Job drawing, mm, ordinate dimensions from the low corner. One solid piece. A direction names the side the tool comes from. Round coordinates to 2 decimals unless told otherwise and drop trailing zeros. Loops run counter-clockwise (first coordinate to the right, second up) from the corner with the lowest first, then second, coordinate; pieces in that order, holes last. Notation, with made-up numbers: M 10,32 L 50,32 A27 cw 50,59 Z; hole C -7.5,-4.5 d2. An arc over 180 degrees is marked long. Use a Markdown table: item, result. Add a question column.
(1) Band-saw the part on A-A, the plane y = 12.25. Write the cut outline in (x, z).
(2) Band-saw the part on B-B, the plane x = 7. Write the cut outline in (y, z) (1 decimal).
(3) Which spindle directions (+Z, -Z, +X, -X, +Y, -Y) get a long thin tool onto all of the face, cutting with end or side? Do the marked faces 1, 2 and 3. Say none if no direction does.
(4) Flat gauge pins, fed straight in: P1, Ø2, axis at y = 2.5, z = 7, coming from the -X side; P2, Ø8, axis at x = 5, y = 6, coming from the -Z side; P3, Ø5, axis at y = 8, z = 11.5, coming from the -X side. Where does each tip first touch, or does it go through?
(5) Band-saw the part on C-C, the plane z = 7. Write the cut outline in (x, y) (1 decimal), and give its area (3 significant figures).
(6) Band-saw the part on D-D, the plane y = 1.5. Write the cut outline in (x, z) (1 decimal), and give its area (3 significant figures).
(7) Wall check: L1, parallel to X at y = 2, z = 7; L2, parallel to Y at x = 9, z = 8.75; L3, parallel to Z at x = 2, y = 2.75 (1 decimal). Give the ranges that are in metal, low to high.
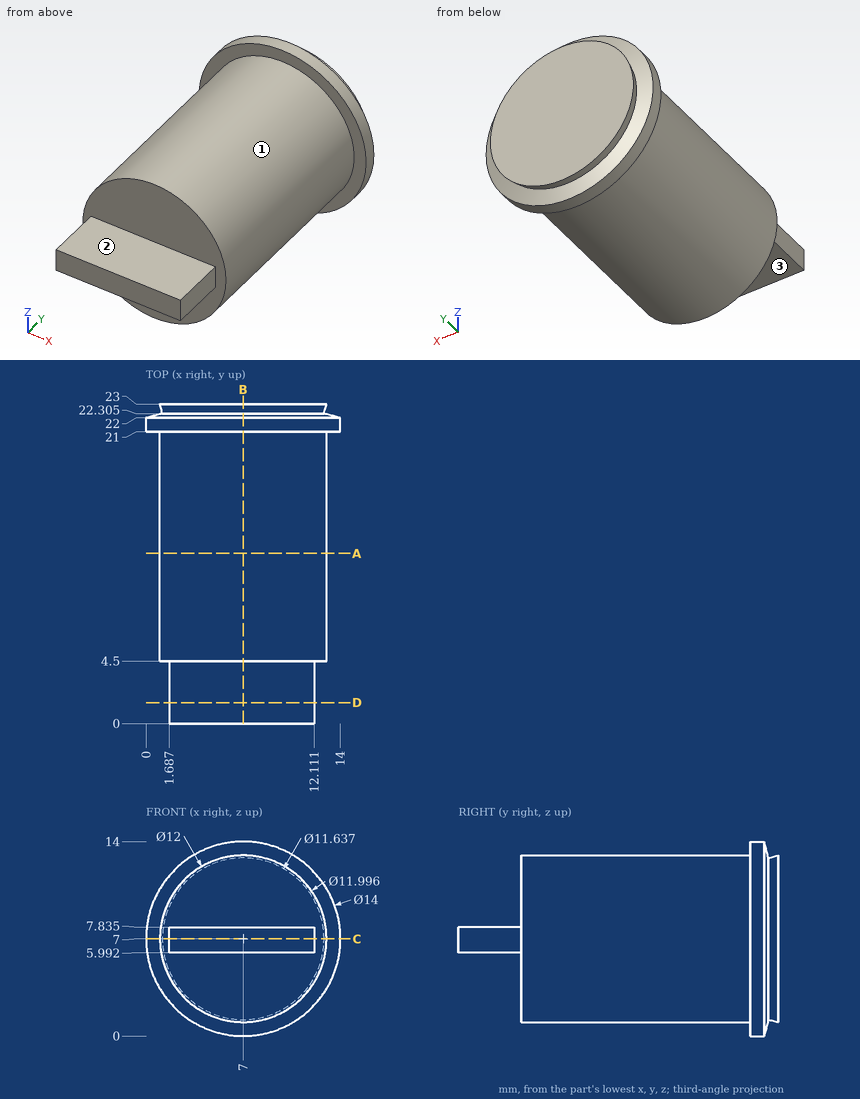
Return value:
| question | item | result |
|---|---|---|
| 1 | outline | C 7,7 d12 |
| 2 | outline | M 0,6 L 4.5,6 L 4.5,1 L 21,1 L 21,0 L 22,0 L 22.3,1.2 L 23,1 L 23,13 L 22.3,12.8 L 22,14 L 21,14 L 21,13 L 4.5,13 L 4.5,7.8 L 0,7.8 Z |
| 3 | face 1 | -Y |
| 3 | face 2 | +Z, +X, -X, -Y |
| 3 | face 3 | -Z, +X, -X, -Y |
| 4 | P1 | x = 1.69 |
| 4 | P2 | z = 1 |
| 4 | P3 | x = 1.34 |
| 5 | outline | M 0,21 L 1,21 L 1,4.5 L 1.7,4.5 L 1.7,0 L 12.1,0 L 12.1,4.5 L 13,4.5 L 13,21 L 14,21 L 14,22 L 12.8,22.3 L 13,23 L 1,23 L 1.2,22.3 L 0,22 Z |
| 5 | area | 271 mm^2 |
| 6 | outline | M 1.7,6 L 12.1,6 L 12.1,7.8 L 1.7,7.8 Z |
| 6 | area | 19.2 mm^2 |
| 7 | L1 | 1.69 to 12.11 |
| 7 | L2 | 4.5 to 23 |
| 7 | L3 | 6 to 7.8 |
